Here's how the part is built. I have some questions about the finished solid (model axes, mm). A direction names the side the tool comes from. Round coordinates to 2 decimals unless told otherwise and drop trailing zeros. Order: outer loops, then holes, each group sorted by start corner. A loop starts at its lowest first (then second) coordinate and runs counter-clockwise, first axis right, second up. Notation, with made-up numbers: (1.25, -8.5) - (37.25, -8.5) arc R5 cw to (37.25, -0.5) - close; hole circle Ø9 at (-32, 81). An arc over 180 degrees is marked (long way). One line per item, written item: value.
from build123d import *

# Parameters (mm, degrees)
F1_DEPTH = 20
F2_R     = 2
F3_R     = 1


with BuildPart() as f1:
    # F0 (on Top) → F1 (new body)
    with BuildSketch(Plane.XY):
        with BuildLine():
            ThreePointArc((1, 0), (0.2928932188, 0.2928932188), (0, 1))
            Line((0, 1), (0, 17.5657877399))
            ThreePointArc((0, 17.5657877399), (1.9080098396, 21.9539099496), (6.4185388425, 23.5511720414))
            Line((6.4185388425, 23.5511720414), (28.3631797552, 22.0166532631))
            ThreePointArc((28.3631797552, 22.0166532631), (29.7669159745, 21.2936816032), (30.208759111, 19.7777864758))
            Line((30.208759111, 19.7777864758), (29.3687820043, 12.9367219271))
            Line((29.3687820043, 12.9367219271), (31.5132220522, 12.7599401181))
            Line((31.5132220522, 12.7599401181), (32.342733337, 19.5157673875))
            ThreePointArc((32.342733337, 19.5157673875), (31.4259088288, 22.6612497768), (28.5131561738, 24.1614159712))
            Line((28.5131561738, 24.1614159712), (28.1860586203, 24.1842888603))
            Line((28.1860586203, 24.1842888603), (26.0360586203, 24.1842888603))
            Line((26.0360586203, 24.1842888603), (26.0360586203, 24.334631506))
            Line((26.0360586203, 24.334631506), (6.568515261, 25.6959347495))
            ThreePointArc((6.568515261, 25.6959347495), (0.4417133655, 23.526320408), (-2.15, 17.5657877399))
            Line((-2.15, 17.5657877399), (-2.15, 1))
            ThreePointArc((-2.15, 1), (-1.2273863607, -1.2273863607), (1, -2.15))
            Line((1, -2.15), (2.2, -2.15))
            ThreePointArc((2.2, -2.15), (4.4273863607, -1.2273863607), (5.35, 1))
            Line((5.35, 1), (5.35, 3.1444985108))
            ThreePointArc((5.35, 3.1444985108), (5.6127226632, 3.8200887184), (6.2628442573, 4.1406932089))
            Line((6.2628442573, 4.1406932089), (7.6935855904, 4.2658668559))
            ThreePointArc((7.6935855904, 4.2658668559), (9.2258107753, 4.8235512154), (10.27391453, 6.0726326305))
            Line((10.27391453, 6.0726326305), (11.7203888097, 9.1746067338))
            Line((11.7203888097, 9.1746067338), (9.7718270676, 10.0832359965))
            Line((9.7718270676, 10.0832359965), (8.3253527878, 6.9812618932))
            ThreePointArc((8.3253527878, 6.9812618932), (7.9926214371, 6.5847281106), (7.5062007435, 6.4076854568))
            Line((7.5062007435, 6.4076854568), (5.9385327718, 6.2705322811))
            ThreePointArc((5.9385327718, 6.2705322811), (3.9881679896, 5.3087188097), (3.2, 3.2819481869))
            Line((3.2, 3.2819481869), (3.2, 1))
            ThreePointArc((3.2, 1), (2.9071067812, 0.2928932188), (2.2, 0))
            Line((2.2, 0), (1, 0))
        make_face()
        Polygon((26.0360586203, 24.1842888603), (28.1860586203, 24.1842888603), (26.0360586203, 24.334631506), align=None)
        Polygon((26.0360586203, 24.334631506), (28.1860586203, 24.1842888603), (28.1860586203, 31.1842888603), (26.0360586203, 31.1842888603), align=None)
    extrude(amount=F1_DEPTH)

    # F2
    f2_edges = [f1.edges().sort_by_distance(p)[0] for p in [
        (27.111059, 31.184289, 20),
        (27.111059, 31.184289, 0),
    ]]
    fillet(f2_edges, radius=F2_R)

    # F3
    f3_edges = [f1.edges().sort_by_distance(p)[0] for p in [
        (26.036059, 24.334632, 10),
        (28.186059, 24.184289, 10),
    ]]
    fillet(f3_edges, radius=F3_R)


solid = f1.part
Q1. If I drill on line 1 along X through (y, z) = (1, 7.75); line 2 along X through (y, z) = (17, 9); line 3 along Y through (x, z) = (1.5, 6.25), over which ranges is the centre line in solid material (lowest first)?
Results list:
line 1: -2.15 to 0, 3.2 to 5.35
line 2: -2.15 to 0, 29.87 to 32.03
line 3: -2.15 to 0, 21.53 to 24.36
Q2. If we section it at B-B, the plane y = 17: Please give me the cut outline in (x, z), then the cut area to 3 significant figures.
Results list:
outline: (-2.15, 0) - (0, 0) - (0, 20) - (-2.15, 20) - close; (29.87, 0) - (32.03, 0) - (32.03, 20) - (29.87, 20) - close
area: 86.3 mm²
Q3. Will these pins go through, and if not, where does the flat tip stop? pin 1 (10 mm diameter, centred on x = 3, z = 4, fed in from +Y); pin 2 (1.1 mm diameter, centred on y = 2, z = 10, fed in from +X); pin 3 (1.5 mm diameter, centred on y = 9.5, z = 17, fed in from +X).
Results list:
pin 1: y = 25.72
pin 2: x = 5.35
pin 3: x = 11.72
Q4. If we section it at D-D, the plane x = 27: Please give me the cut outline in (y, z), then the cut area to 3 significant figures.
Results list:
outline: (22.11, 0) - (29.18, 0) arc R2 ccw to (31.18, 2) - (31.18, 18) arc R2 ccw to (29.18, 20) - (22.11, 20) - close
area: 180 mm²
Q5. Which directions (+Z, -Z, +X, -X, +Y, -Y) give clear straight access to the entire face, cutting with the end or side of a thin tool? Please do faces 4 (the flat face through (15.896, 25.044, 9.86)), 5 (the flat face through (10.76, 9.623, 9.86)), 6 (the flat face through (9.059, 8.554, 9.86)).
Results list:
face 4: +Z, -Z, +Y
face 5: +Z, -Z, +X
face 6: +Z, -Z
Q6. If we section it at A-A, the plane x = 7: Please give me the cut outline in (y, z).
Results list:
outline: (4.21, 0) - (6.36, 0) - (6.36, 20) - (4.21, 20) - close; (23.51, 0) - (25.67, 0) - (25.67, 20) - (23.51, 20) - close
Q7. If we section it at C-C, the plane y = 28.5: Please give me the cut outline in (x, z).
Results list:
outline: (26.04, 0) - (28.19, 0) - (28.19, 20) - (26.04, 20) - close
Q8. We'd pull the mould along Y, two halves only. Please class faces 1 (the cylindrical face through (1, 24, 10)), 2 (the cylindrical face through (1.86, 21.91, 9.86)), 3 (the flat face through (11, 9, 20)): released by +Y, released by -Y, zero draft, split by the parting line, or undercut.
Results list:
face 1: released by +Y
face 2: undercut
face 3: zero draft
